Design review of the part shown in the three views and the two pictorial views. Dimensions are in mm from the part's minimum x, y and z. Give positions to 0.01 mm unless a question says otherwise; leave off trailing zeros. Order: outer loops, then holes, each group sorted by start corner. A loop starts at its lowest first (then second) coordinate and runs counter-clockwise, first axis right, second up. Notation, with made-up numbers: (23, 73.5) -> (60, 73.5) arc R19 ccw to (60, 78.5) -> close; hole circle Ø5 at (-40, 54). An arc over 180 degrees is marked (long way). Answer in a Markdown table with one row per item. Add a question column.
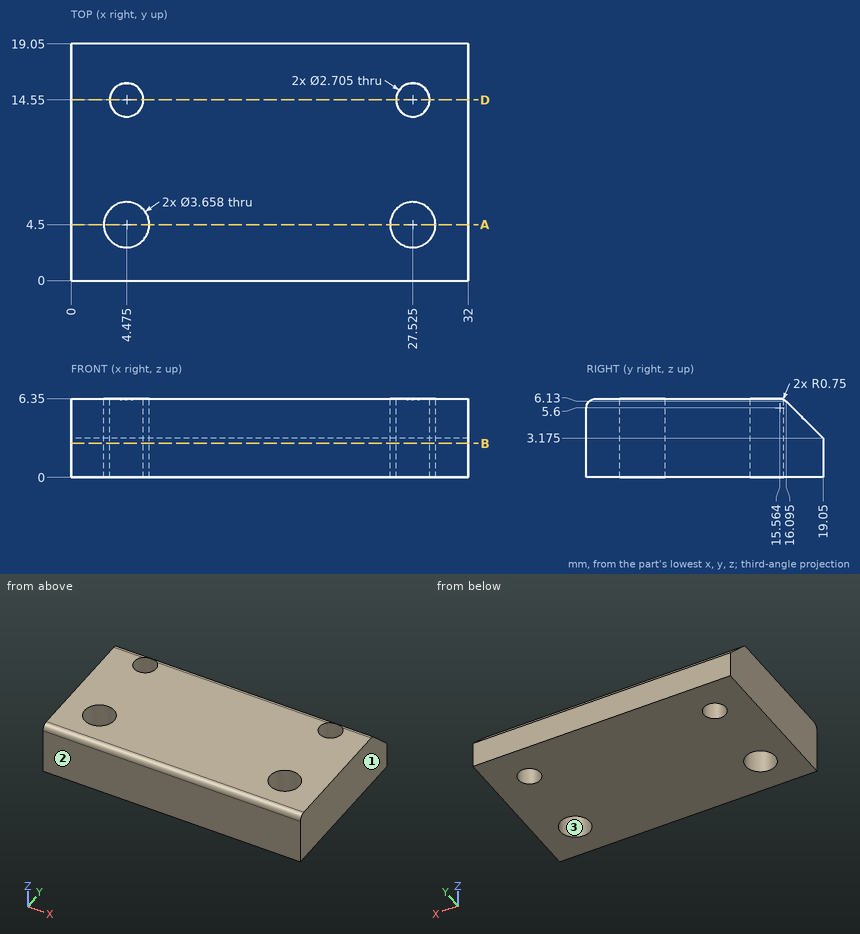
1) Add section D-D, the plane y = 14.55. Write out the cut boundary in (x, z).
2) Mouldability with a two-part tool opening along X and no side actions: class the marked faces 1, 2 and 3 as +X half, -X half, draft (parallel to the pull), parting line (faces both ways), or undercut.
3) Add section B-B, the plane z = 2.75. Give the number of separate pieces and of enclosed holes in the cut face, and give its area (3 significant figures).
4) For L1, parallel to Y at x = 27.5, z = 0.5; L2, parallel to X at y = 14.55, z = 1.5; L3, parallel to Y at x = 5.5, z = 3.25 (1 decimal), list the stretches that pass through material, from the lowest coordinate up.
5) Add section A-A, the plane y = 4.5. Write out the cut boundary in (x, z), and give its area (3 significant figures).
Verdict:
| question | item | result |
|---|---|---|
| 1 | outline | (0, 0) -> (3.12, 0) -> (3.12, 6.35) -> (0, 6.35) -> close; (5.83, 0) -> (26.17, 0) -> (26.17, 6.35) -> (5.83, 6.35) -> close; (28.88, 0) -> (32, 0) -> (32, 6.35) -> (28.88, 6.35) -> close |
| 2 | face 1 | +X half |
| 2 | face 2 | draft |
| 2 | face 3 | undercut |
| 3 | separate pieces | 1 |
| 3 | enclosed holes | 4 |
| 3 | area | 577 mm2 |
| 4 | L1 | y = 0 to 2.67, 6.33 to 13.2, 15.9 to 19.05 |
| 4 | L2 | x = 0 to 3.12, 5.83 to 26.17, 28.88 to 32 |
| 4 | L3 | y = 0 to 3, 6 to 13.7, 15.4 to 19 |
| 5 | outline | (0, 0) -> (2.65, 0) -> (2.65, 6.35) -> (0, 6.35) -> close; (6.3, 0) -> (25.7, 0) -> (25.7, 6.35) -> (6.3, 6.35) -> close; (29.35, 0) -> (32, 0) -> (32, 6.35) -> (29.35, 6.35) -> close |
| 5 | area | 157 mm2 |
